from build123d import *

# Parameters (mm, degrees)
F0_R     = 11
F0_R_2   = 4.75
F0_R_3   = 4.2
F1_DEPTH = 1.5
F2_DEPTH = 3.6
F3_R     = 1
F4_R     = 0.5
F5_DEPTH = 0.6


with BuildPart() as f1:
    # F0 (on Top) → F1 (new body)
    with BuildSketch(Plane.XY):
        Circle(F0_R)
        Circle(F0_R_2, mode=Mode.SUBTRACT)
        Circle(F0_R_2)
        Circle(F0_R_3, mode=Mode.SUBTRACT)
        Circle(F0_R_3)
    extrude(amount=-F1_DEPTH)

    # F0 (on Top) → F2 (join)
    with BuildSketch(Plane.XY):
        Circle(F0_R_3)
    extrude(amount=F2_DEPTH)

    # F3
    f3_edges = [f1.edges().sort_by_distance(p)[0] for p in [
        (-11, 0, 0),
    ]]
    fillet(f3_edges, radius=F3_R)

    # F4
    f4_edges = [f1.edges().sort_by_distance(p)[0] for p in [
        (-4.2, 0, 3.6),
    ]]
    fillet(f4_edges, radius=F4_R)

    # F0 (on Top) → F5 (join)
    with BuildSketch(Plane.XY):
        Circle(F0_R_2)
        Circle(F0_R_3, mode=Mode.SUBTRACT)
    extrude(amount=F5_DEPTH)


solid = f1.part
Check sheet for the modelled part. Datum: model origin and axes. Units: mm. A direction names the side the tool comes from. Give positions to 0.01 mm unless a question says otherwise; leave off trailing zeros. Write each loop counter-clockwise with the first axis right and the second up, starting at its lowest first coordinate (ties: lowest second). Pieces come first, ordered by that corner, then holes. Notation, with made-up numbers: M 50,-23.5 L 108,-23.5 A26 ccw 108,-2.5 Z; hole C -4.75,14 d9. An arc over 180 degrees is marked long. Use one line per item in the form item = value.
(1) Material ranges on line 1 along Z through (x, y) = (1.75, 4); line 2 along Z through (x, y) = (-4.5, -3.25); line 3 along Y through (x, z) = (-3.5, 0.4), recorded low to high.
Answer block:
line_1 = -1.5 to 0.6
line_2 = -1.5 to 0
line_3 = -3.21 to 3.21
(2) Depth check by flat-ended pin: P1, Ø1, axis at y = -3, z = 1, coming from the -X side; P2, Ø1, axis at x = -8.5, z = 1.5, coming from the +Y side. Enter the tip coordinate at first touch or a pass-through.
Answer block:
P1 = -3.91
P2 = through
(3) Section check A-A on x = 0. Record the boundary of the cut face in (y, z), plus the area to 3 significant figures.
Answer block:
outline = M -11,-1.5 L 11,-1.5 L 11,-1 A1 ccw 10,0 L 4.75,0 L 4.75,0.6 L 4.2,0.6 L 4.2,3.1 A0.5 ccw 3.7,3.6 L -3.7,3.6 A0.5 ccw -4.2,3.1 L -4.2,0.6 L -4.75,0.6 L -4.75,0 L -10,0 A1 ccw -11,-1 Z
area = 63.4 mm2
(4) Tool access check on faces 1 (the cylindrical face through (-2.38, -10.74, -1.25)), 2 (the cylindrical face through (4.006, 1.262, 1.832)). Record the directions out of +Z, -Z, +X, -X, +Y, -Y that give a thin tool (end or side, any length) a straight path to the whole face; none if there is none.
Answer block:
face_1 = +Z, -Z
face_2 = +Z
